Could you check a few things on this model? Use its own coordinates, in mm. Face numbers are marked on the shaded views. A direction names the side the tool comes from. Coordinates: 2 decimals unless noted, no trailing zeros. Write each loop counter-clockwise with the first axis right and the second up, starting at its lowest first coordinate (ties: lowest second). Pieces come first, ordered by that corner, then holes. Notation, with made-up numbers: (-20, -0.75) - (36, -0.75) arc R33 ccw to (36, 31.25) - close; hole circle Ø1 at (-28, 2.5). An arc over 180 degrees is marked (long way). Answer as a JSON object with one key per item and string values. Group by question number.
1) Please list where these lines run through material, in increasing order: line 1 along X through (y, z) = (-5, 3.5); line 2 along Y through (x, z) = (11, 4.75); line 3 along Y through (x, z) = (10.5, 1).
2) If we section it at D-D (y = 1.75): Write out the boundary of the cut face in (x, z).
3) Will these pins go through, and if not, where does the flat tip stop? pin 1 Ø4 at (x, y) = (-10.5, 6.5) entering from -Z; pin 2 Ø1.5 at (x, y) = (7.5, 4) entering from -Z; pin 3 Ø2.5 at (y, z) = (3, 6.5) entering from -X; pin 4 Ø4 at (x, z) = (-1.5, 3) entering from +Y.
4) If we section it at A-A (y = 5): Write out the boundary of the cut face in (x, z), plus the area to 3 significant figures.
5) We'd pull the mould along X, two halves only. Please class the marked faces 3, 4 and 5: released by +X, released by -X, zero draft, split by the parting line, or undercut.
6) If we section it at C-C (x = 3.5): Write out the boundary of the cut face in (y, z).
7) If we section it at B-B (z = 13.5): Write out the boundary of the cut face in (x, y), plus the area to 3 significant figures.
8) On a 3-axis mill with a long thin cutter (end or side, diameter ignored), from which of +Z, -Z, +X, -X, +Y, -Y can I reach the whole of each face in a straight line? I mean the marked faces 1 and 2. Say none if no direction works.
```python
from build123d import *

# Parameters (mm, degrees)
ESQUISSE1_W             = 30
ESQUISSE1_H             = 20
ESQUISSE1_R             = 2.5
BOSS_EXTRU_1_DEPTH      = 15
ESQUISSE2_W             = 19.552131663
ESQUISSE2_H             = 8.703273887
ENL_V_MAT_EXTRU_1_DEPTH = 11


with BuildPart() as part:
    # Esquisse1 → Boss.-Extru.1 (new body)
    with BuildSketch(Plane.XY):
        Rectangle(ESQUISSE1_W, ESQUISSE1_H)
        with Locations((9.763813692, 5)):
            Circle(ESQUISSE1_R, mode=Mode.SUBTRACT)
        with Locations(Location((9.763813692, -5, 0), (0, 0, 180))):
            Circle(ESQUISSE1_R, mode=Mode.SUBTRACT)
    extrude(amount=BOSS_EXTRU_1_DEPTH)

    # Esquisse2 → Enlèv. mat.-Extru.1 (cut)
    with BuildSketch(Plane(origin=(0, 10, 0), x_dir=(1, 0, 0), z_dir=(0, 1, 0))):
        with Locations((-5.223934169, -4.351636943)):
            Rectangle(ESQUISSE2_W, ESQUISSE2_H)
    extrude(amount=-ENL_V_MAT_EXTRU_1_DEPTH, mode=Mode.SUBTRACT)


solid = part.part
```
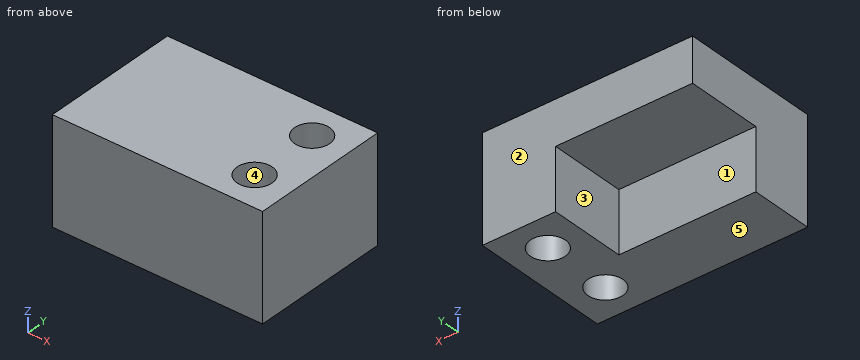
Here are the results:
{
 "1": {"line 1": "x = -15 to 7.26, 12.26 to 15", "line 2": "y = -10 to -7.17, -2.83 to 2.83, 7.17 to 10", "line 3": "y = -10 to -7.39, -2.61 to 2.61, 7.39 to 10"},
 "2": {"outline": "(-15, 8.7) - (4.55, 8.7) - (4.55, 0) - (15, 0) - (15, 15) - (-15, 15) - close"},
 "3": {"pin 1": "stops at z = 8.7", "pin 2": "stops at z = 0", "pin 3": "stops at x = 4.55", "pin 4": "stops at y = -1"},
 "4": {"outline": "(-15, 8.7) - (4.55, 8.7) - (4.55, 0) - (7.26, 0) - (7.26, 15) - (-15, 15) - close; (12.26, 0) - (15, 0) - (15, 15) - (12.26, 15) - close", "area": "205 mm²"},
 "5": {"face 3": "released by -X", "face 4": "undercut", "face 5": "zero draft"},
 "6": {"outline": "(-10, 0) - (-1, 0) - (-1, 8.7) - (10, 8.7) - (10, 15) - (-10, 15) - close"},
 "7": {"outline": "(-15, -10) - (15, -10) - (15, 10) - (-15, 10) - close; hole circle Ø5 at (9.76, -5); hole circle Ø5 at (9.76, 5)", "area": "561 mm²"},
 "8": {"face 1": "-Z, -X, +Y", "face 2": "+Z, -Z, +X, -X, +Y"}
}
